Source: three-view drawing plus pictorial views. Frame: mm from the lowest corner of the part. A direction names the side the tool comes from. Coordinates: 2 decimals unless noted, no trailing zeros. Loops run counter-clockwise (first coordinate to the right, second up) from the corner with the lowest first, then second, coordinate; pieces in that order, holes last. Notation, with made-up numbers: (-40, -31) - (2, -31) arc R31 ccw to (2, 4) - close; hole circle Ø1 at (74.25, 24). An arc over 180 degrees is marked (long way). Answer as CSV lines item,"result". Start each with the question number.
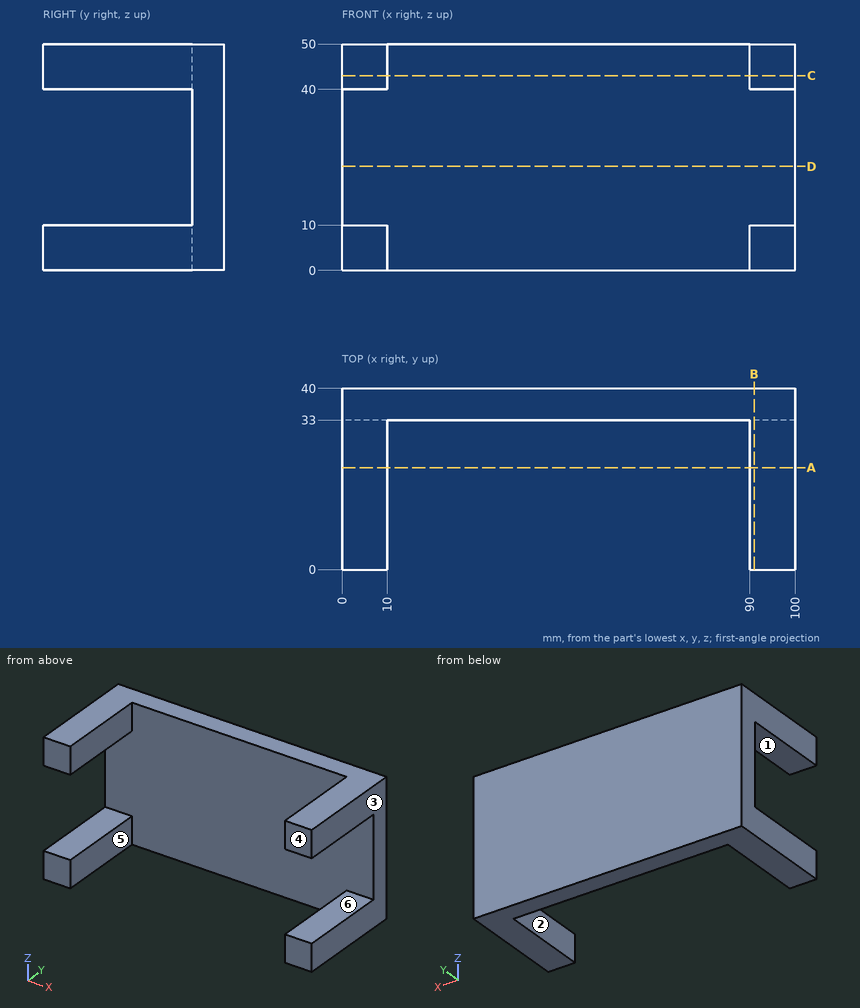
Item 1: Section query D-D, the plane z = 23. Output: boundary loops of the cut face in (x, y), and give its area (3 significant figures).
Item 2: Section query C-C, the plane z = 43. Output: boundary loops of the cut face in (x, y).
Item 3: Contact query for a flat-ended pin moving along its axis: P1, Ø8, axis at x = 83, z = 16, coming from the -Y side. Output: stop coordinate, or through.
Item 4: Set-up query: the marked faces 4, 5 and 6. Return all of +Z, -Z, +X, -X, +Y, -Y with unobstructed straight access to the full face (end or side cutting, diameter ignored); none if empty.
Item 5: Section query B-B, the plane x = 91. Output: boundary loops of the cut face in (y, z).
Item 6: Section query A-A, the plane y = 22.5. Output: boundary loops of the cut face in (x, z).
Item 7: Draft query along X for the marked faces 1, 2 and 3. Return one class per face: pulls with the +X half, pulls with the -X half, needs draft (parallel to the pull), parting line crosses it, or undercut.
Item 8: Material intervals for probe 1 along Y at (x, z) = (27, 43); probe 2 along X at (y, z) = (18, 41), sorted ascending.
Response values:
1,outline,"(0, 33) - (100, 33) - (100, 40) - (0, 40) - close"
1,area,"700 mm²"
2,outline,"(0, 0) - (10, 0) - (10, 33) - (90, 33) - (90, 0) - (100, 0) - (100, 40) - (0, 40) - close"
3,P1,"stops at y = 33"
4,face 4,"+Z, -Z, +X, -X, -Y"
4,face 5,"+Z, -Z, -Y"
4,face 6,"+X, -X, -Y"
5,outline,"(0, 0) - (40, 0) - (40, 50) - (0, 50) - (0, 40) - (33, 40) - (33, 10) - (0, 10) - close"
6,outline,"(0, 0) - (10, 0) - (10, 10) - (0, 10) - close; (0, 40) - (10, 40) - (10, 50) - (0, 50) - close; (90, 0) - (100, 0) - (100, 10) - (90, 10) - close; (90, 40) - (100, 40) - (100, 50) - (90, 50) - close"
7,face 1,"needs draft"
7,face 2,"undercut"
7,face 3,"pulls with the +X half"
8,probe 1,"y = 33 to 40"
8,probe 2,"x = 0 to 10, 90 to 100"
